```python
from build123d import *

# Parameters (mm, degrees)
SKETCH1_W           = 95
SKETCH1_H           = 24
BOSS_EXTRUDE1_DEPTH = 27
SKETCH2_W           = 17
SKETCH2_H           = 12.4
CUT_EXTRUDE1_DEPTH  = 56.939699677
SKETCH3_W           = 80
SKETCH3_H           = 44.068449986
CUT_EXTRUDE2_DEPTH  = 20
SKETCH4_W           = 24
SKETCH4_H           = 3
BOSS_EXTRUDE2_DEPTH = 6
SKETCH5_W           = 24
SKETCH5_H           = 3
BOSS_EXTRUDE3_DEPTH = 6
SKETCH6_R           = 1.25
CUT_EXTRUDE3_DEPTH  = 60.851900555
SKETCH7_R           = 1.25
CUT_EXTRUDE4_DEPTH  = 60.851900555


with BuildPart() as part:
    # Sketch1 → Boss-Extrude1 (new body)
    with BuildSketch(Plane(origin=(0, 0, 0), x_dir=(1, 0, 0), z_dir=(0, 1, 0))):
        Rectangle(SKETCH1_W, SKETCH1_H)
    extrude(amount=BOSS_EXTRUDE1_DEPTH)

    # Sketch2 → Cut-Extrude1 (cut, through all)
    with BuildSketch(Plane(origin=(0, 27, 0), x_dir=(1, 0, 0), z_dir=(0, 1, 0))):
        with Locations((19.1, 0)):
            Rectangle(SKETCH2_W, SKETCH2_H)
        Rectangle(SKETCH2_W, SKETCH2_H)
        with Locations((-19.1, 0)):
            Rectangle(SKETCH2_W, SKETCH2_H)
        with Locations((-38.2, 0)):
            Rectangle(SKETCH2_W, SKETCH2_H)
        with Locations((38.2, 0)):
            Rectangle(SKETCH2_W, SKETCH2_H)
    extrude(amount=-CUT_EXTRUDE1_DEPTH, mode=Mode.SUBTRACT)

    # Sketch3 → Cut-Extrude2 (cut)
    with BuildSketch(Plane.XZ):
        Rectangle(SKETCH3_W, SKETCH3_H)
    extrude(amount=-CUT_EXTRUDE2_DEPTH, mode=Mode.SUBTRACT)

    # Sketch4 → Boss-Extrude2 (add)
    with BuildSketch(Plane(origin=(47.5, 0, 0), x_dir=(0, 0, -1), z_dir=(1, 0, 0))):
        with Locations((0, 1.5)):
            Rectangle(SKETCH4_W, SKETCH4_H)
    extrude(amount=BOSS_EXTRUDE2_DEPTH)

    # Sketch5 → Boss-Extrude3 (add)
    with BuildSketch(Plane.ZY.offset(47.5)):
        with Locations((0, 1.5)):
            Rectangle(SKETCH5_W, SKETCH5_H)
    extrude(amount=BOSS_EXTRUDE3_DEPTH)

    # Sketch6 → Cut-Extrude3 (cut, through all)
    with BuildSketch(Plane(origin=(0, 3, 0), x_dir=(1, 0, 0), z_dir=(0, 1, 0))):
        with Locations(Location((50.45345714, -0.537948729, 0), (0, 0, 270))):
            Circle(SKETCH6_R)
    extrude(amount=-CUT_EXTRUDE3_DEPTH, mode=Mode.SUBTRACT)

    # Sketch7 → Cut-Extrude4 (cut, through all)
    with BuildSketch(Plane(origin=(0, 3, 0), x_dir=(1, 0, 0), z_dir=(0, 1, 0))):
        with Locations(Location((-50.910758479, 0.436684104, 0), (0, 0, 270))):
            Circle(SKETCH7_R)
    extrude(amount=-CUT_EXTRUDE4_DEPTH, mode=Mode.SUBTRACT)


solid = part.part
```
The listing builds one solid part. Answer for the finished solid, in the listing's coordinates (mm). A direction names the side the tool comes from. Give positions to 0.01 mm unless a question says otherwise; leave off trailing zeros. Order: outer loops, then holes, each group sorted by start corner. A loop starts at its lowest first (then second) coordinate and runs counter-clockwise, first axis right, second up. Notation, with made-up numbers: M -37.75,37 L -14.75,37 A28 ccw -14.75,66 Z; hole C -21,63.25 d8. An arc over 180 degrees is marked long. Put each result on its own line as item: value. Start each with the question number.
Item 1: For a pull along Z with two mould halves and no side action, classify faces 5 (the face through (0, 22, -12)), 6 (the face through (49, 3, 0)), 7 (the face through (8.5, 24, 0)) as +Z half, -Z half, draft (parallel to the pull), parting line (faces both ways), or undercut.
Item 2: Find the intervals of material crossed by line 1 along X through (y, z) = (23, -5.5); line 2 along X through (y, z) = (7.25, -6); line 3 along Z through (x, y) = (-43, 15.25), in increasing order.
Item 3: The part is cut by section A-A, the plane x = 3. Determine the outline of the cut face in (y, z), and give its area (3 significant figures).
Item 4: Flat-ended cylindrical pins translate along their axes: P1, Ø2, axis at y = 18.5, z = 5, coming from the -X side; P2, Ø3, axis at x = 50.45, z = 0.54, coming from the +Y side; P3, Ø3, axis at y = 8, z = 9.5, coming from the +X side; P4, Ø5, axis at x = -39, y = 12, coming from the -Z side. Find the tip coordinate at first contact, or state that the pin passes through.
Item 5: Which of the six approach directions +Z, -Z, +X, -X, +Y, -Y give full straight-line access (tool end or side, diameter ignored) to faces 1 (the face through (-19, 24, -6.2)), 2 (the face through (53.5, 2, 0)), 3 (the face through (-49, 3, 0)), 4 (the face through (-40, 10, 9))?
Item 6: The part is cut by section D-D, the plane z = -8.5. Determine the outline of the cut face in (x, y).
Item 7: The part is cut by section B-B, the plane z = 2.75. Determine the outline of the cut face in (x, y).
Item 8: The part is cut by section C-C, the plane y = 12.5. Determine the outline of the cut face in (x, z).
Answer key:
1. face 5: -Z half
1. face 6: draft
1. face 7: undercut
2. line 1: x = -47.5 to -46.7, -29.7 to -27.6, -10.6 to -8.5, 8.5 to 10.6, 27.6 to 29.7, 46.7 to 47.5
2. line 2: x = -47.5 to -46.7, 46.7 to 47.5
2. line 3: z = -12 to -6.2, 6.2 to 12
3. outline: M 20,-12 L 27,-12 L 27,-6.2 L 20,-6.2 Z; M 20,6.2 L 27,6.2 L 27,12 L 20,12 Z
3. area: 81.2 mm²
4. P1: stops at x = -47.5
4. P2: stops at y = 3
4. P3: stops at x = 47.5
4. P4: stops at z = -12
5. face 1: +Y, -Y
5. face 2: +Z, -Z, +X, +Y, -Y
5. face 3: +Z, -Z, -X, +Y
5. face 4: +Z, -Z, -Y
6. outline: M -53.5,0 L -40,0 L -40,20 L 40,20 L 40,0 L 53.5,0 L 53.5,3 L 47.5,3 L 47.5,27 L -47.5,27 L -47.5,3 L -53.5,3 Z
7. outline: M -53.5,0 L -46.7,0 L -46.7,27 L -47.5,27 L -47.5,3 L -53.5,3 Z; M -29.7,20 L -27.6,20 L -27.6,27 L -29.7,27 Z; M -10.6,20 L -8.5,20 L -8.5,27 L -10.6,27 Z; M 8.5,20 L 10.6,20 L 10.6,27 L 8.5,27 Z; M 27.6,20 L 29.7,20 L 29.7,27 L 27.6,27 Z; M 46.7,0 L 53.5,0 L 53.5,3 L 47.5,3 L 47.5,27 L 46.7,27 Z
8. outline: M -47.5,-12 L -40,-12 L -40,-6.2 L -46.7,-6.2 L -46.7,6.2 L -40,6.2 L -40,12 L -47.5,12 Z; M 40,-12 L 47.5,-12 L 47.5,12 L 40,12 L 40,6.2 L 46.7,6.2 L 46.7,-6.2 L 40,-6.2 Z
